```python
from build123d import *

# Parameters (mm, degrees)
SKETCH_1_W                    = 38
SKETCH_1_H                    = 78
EXTRUDE_1_DEPTH               = 7.8
SKETCH_3_W                    = 38
SKETCH_3_H                    = 7.8
EXTRUDE_2_DEPTH               = 78
EXTRUDE_3_DEPTH               = 3.8
SKETCH_5_R                    = 4.25
CUT_EXTRUDE_1_DEPTH           = 102.079572615
SKETCH_6_W                    = 8.8
SKETCH_6_H                    = 70
CUT_EXTRUDE_2_DEPTH           = 4
CUT_EXTRUDE_2_DRAFT           = -2
CUT_EXTRUDE_2_PROFILE_2_DEPTH = 4
CUT_EXTRUDE_2_PROFILE_2_DRAFT = -2
CUT_EXTRUDE_2_PROFILE_3_DEPTH = 4
CUT_EXTRUDE_2_PROFILE_3_DRAFT = -2
SKETCH_7_W                    = 8.8
SKETCH_7_H                    = 70
CUT_EXTRUDE_3_DEPTH           = 4
CUT_EXTRUDE_3_DRAFT           = -2
CUT_EXTRUDE_3_PROFILE_2_DEPTH = 4
CUT_EXTRUDE_3_PROFILE_2_DRAFT = -2
CUT_EXTRUDE_3_PROFILE_3_DEPTH = 4
CUT_EXTRUDE_3_PROFILE_3_DRAFT = -2


with BuildPart() as part:
    # 草图1 → 凸台-拉伸1 (new body)
    with BuildSketch(Plane.XY):
        Rectangle(SKETCH_1_W, SKETCH_1_H)
    extrude(amount=EXTRUDE_1_DEPTH)

    # 草图3 → 凸台-拉伸2 (add)
    with BuildSketch(Plane.XY.offset(7.8)):
        with Locations((0, -35.1)):
            Rectangle(SKETCH_3_W, SKETCH_3_H)
    extrude(amount=-EXTRUDE_2_DEPTH)

    # 草图4 → 凸台-拉伸3 (add)
    with BuildSketch(Plane.ZY.offset(19)):
        Polygon((0, 39), (-7.8, 39), (-7.8, 34), (-65.2, -23.4), (-70.2, -23.4), (-70.2, -31.2), (0, -31.2), align=None)
    extrude(amount=-EXTRUDE_3_DEPTH)

    # 草图5 → 切除-拉伸1 (cut, through all)
    with BuildSketch(Plane(origin=(0, -31.2, 0), x_dir=(1, 0, 0), z_dir=(0, 1, 0))):
        with Locations(Location((0, 54.416495981, 0), (0, 0, 270))):
            Circle(SKETCH_5_R)
        with BuildLine():
            Line((-4.1430597, 19.083232121), (-4.1430597, 36.583232121))
            ThreePointArc((-4.1430597, 36.583232121), (0, 40.726291822), (4.1430597, 36.583232121))
            Line((4.1430597, 36.583232121), (4.1430597, 19.083232121))
            ThreePointArc((4.1430597, 19.083232121), (0, 14.940172421), (-4.1430597, 19.083232121))
        make_face()
    cut_extrude_1 = extrude(amount=-CUT_EXTRUDE_1_DEPTH, mode=Mode.SUBTRACT)

    # 镜向1: 切除-拉伸1 across plane
    add(cut_extrude_1.mirror(Plane(origin=(0, -15.6, -15.6), x_dir=(0, -0.7071067811865478, 0.7071067811865474), z_dir=(0, 0.7071067811865472, 0.7071067811865478))), mode=Mode.SUBTRACT)


with BuildPart() as cut_extrude_2_tool:
    # 草图6 → 切除-拉伸2 (with draft: the straight prism first)
    with BuildSketch(Plane.XZ.offset(39)):
        with Locations((-11.8, -31.2)):
            Rectangle(SKETCH_6_W, SKETCH_6_H)
    extrude(amount=-CUT_EXTRUDE_2_DEPTH)
    # 切除-拉伸2: the draft: its side faces are tilted about the plane it starts from
    cut_extrude_2_sides = [cut_extrude_2_tool.faces().sort_by_distance(p)[0] for p in [
        (-16.2, -37, -31.2),
        (-11.8, -37, -66.2),
        (-7.4, -37, -31.2),
        (-11.8, -37, 3.8),
    ]]
    draft(cut_extrude_2_sides, Plane.XZ.offset(39), CUT_EXTRUDE_2_DRAFT)


with BuildPart() as part_1:
    add(part.part)

    # 切除-拉伸2: cut by cut_extrude_2_tool
    add(cut_extrude_2_tool.part, mode=Mode.SUBTRACT)


with BuildPart() as cut_extrude_2_profile_2_tool:
    # 草图6 → 切除-拉伸2 profile 2 (with draft: the straight prism first)
    with BuildSketch(Plane.XZ.offset(39)):
        with Locations((0, -31.2)):
            Rectangle(SKETCH_6_W, SKETCH_6_H)
    extrude(amount=-CUT_EXTRUDE_2_PROFILE_2_DEPTH)
    # 切除-拉伸2 profile 2: the draft: its side faces are tilted about the plane it starts from
    cut_extrude_2_profile_2_sides = [cut_extrude_2_profile_2_tool.faces().sort_by_distance(p)[0] for p in [
        (-4.4, -37, -31.2),
        (0, -37, -66.2),
        (4.4, -37, -31.2),
        (0, -37, 3.8),
    ]]
    draft(cut_extrude_2_profile_2_sides, Plane.XZ.offset(39), CUT_EXTRUDE_2_PROFILE_2_DRAFT)


with BuildPart() as part_2:
    add(part_1.part)

    # 切除-拉伸2 profile 2: cut by cut_extrude_2_profile_2_tool
    add(cut_extrude_2_profile_2_tool.part, mode=Mode.SUBTRACT)


with BuildPart() as cut_extrude_2_profile_3_tool:
    # 草图6 → 切除-拉伸2 profile 3 (with draft: the straight prism first)
    with BuildSketch(Plane.XZ.offset(39)):
        with Locations((11.8, -31.2)):
            Rectangle(SKETCH_6_W, SKETCH_6_H)
    extrude(amount=-CUT_EXTRUDE_2_PROFILE_3_DEPTH)
    # 切除-拉伸2 profile 3: the draft: its side faces are tilted about the plane it starts from
    cut_extrude_2_profile_3_sides = [cut_extrude_2_profile_3_tool.faces().sort_by_distance(p)[0] for p in [
        (7.4, -37, -31.2),
        (11.8, -37, -66.2),
        (16.2, -37, -31.2),
        (11.8, -37, 3.8),
    ]]
    draft(cut_extrude_2_profile_3_sides, Plane.XZ.offset(39), CUT_EXTRUDE_2_PROFILE_3_DRAFT)


with BuildPart() as part_3:
    add(part_2.part)

    # 切除-拉伸2 profile 3: cut by cut_extrude_2_profile_3_tool
    add(cut_extrude_2_profile_3_tool.part, mode=Mode.SUBTRACT)


with BuildPart() as cut_extrude_3_tool:
    # 草图7 → 切除-拉伸3 (with draft: the straight prism first)
    with BuildSketch(Plane.XY.offset(7.8)):
        Rectangle(SKETCH_7_W, SKETCH_7_H)
    extrude(amount=-CUT_EXTRUDE_3_DEPTH)
    # 切除-拉伸3: the draft: its side faces are tilted about the plane it starts from
    cut_extrude_3_sides = [cut_extrude_3_tool.faces().sort_by_distance(p)[0] for p in [
        (-4.4, 0, 5.8),
        (0, -35, 5.8),
        (4.4, 0, 5.8),
        (0, 35, 5.8),
    ]]
    draft(cut_extrude_3_sides, Plane.XY.offset(7.8), CUT_EXTRUDE_3_DRAFT)


with BuildPart() as part_4:
    add(part_3.part)

    # 切除-拉伸3: cut by cut_extrude_3_tool
    add(cut_extrude_3_tool.part, mode=Mode.SUBTRACT)


with BuildPart() as cut_extrude_3_profile_2_tool:
    # 草图7 → 切除-拉伸3 profile 2 (with draft: the straight prism first)
    with BuildSketch(Plane.XY.offset(7.8)):
        with Locations((-11.8, 0)):
            Rectangle(SKETCH_7_W, SKETCH_7_H)
    extrude(amount=-CUT_EXTRUDE_3_PROFILE_2_DEPTH)
    # 切除-拉伸3 profile 2: the draft: its side faces are tilted about the plane it starts from
    cut_extrude_3_profile_2_sides = [cut_extrude_3_profile_2_tool.faces().sort_by_distance(p)[0] for p in [
        (-16.2, 0, 5.8),
        (-11.8, -35, 5.8),
        (-7.4, 0, 5.8),
        (-11.8, 35, 5.8),
    ]]
    draft(cut_extrude_3_profile_2_sides, Plane.XY.offset(7.8), CUT_EXTRUDE_3_PROFILE_2_DRAFT)


with BuildPart() as part_5:
    add(part_4.part)

    # 切除-拉伸3 profile 2: cut by cut_extrude_3_profile_2_tool
    add(cut_extrude_3_profile_2_tool.part, mode=Mode.SUBTRACT)


with BuildPart() as cut_extrude_3_profile_3_tool:
    # 草图7 → 切除-拉伸3 profile 3 (with draft: the straight prism first)
    with BuildSketch(Plane.XY.offset(7.8)):
        with Locations((11.8, 0)):
            Rectangle(SKETCH_7_W, SKETCH_7_H)
    extrude(amount=-CUT_EXTRUDE_3_PROFILE_3_DEPTH)
    # 切除-拉伸3 profile 3: the draft: its side faces are tilted about the plane it starts from
    cut_extrude_3_profile_3_sides = [cut_extrude_3_profile_3_tool.faces().sort_by_distance(p)[0] for p in [
        (7.4, 0, 5.8),
        (11.8, -35, 5.8),
        (16.2, 0, 5.8),
        (11.8, 35, 5.8),
    ]]
    draft(cut_extrude_3_profile_3_sides, Plane.XY.offset(7.8), CUT_EXTRUDE_3_PROFILE_3_DRAFT)


with BuildPart() as part_6:
    add(part_5.part)

    # 切除-拉伸3 profile 3: cut by cut_extrude_3_profile_3_tool
    add(cut_extrude_3_profile_3_tool.part, mode=Mode.SUBTRACT)


solid = part_6.part
```
Part model, mm, in its own coordinate system. A direction names the side the tool comes from. Coordinates: 2 decimals unless noted, no trailing zeros. Write each loop counter-clockwise with the first axis right and the second up, starting at its lowest first coordinate (ties: lowest second). Pieces come first, ordered by that corner, then holes.
Item 1: Slice it at A-A (x = 0). Count the separate pieces of the cut face and the enclosed holes in it, and give its area (3 significant figures).
Item 2: Which spindle directions (+Z, -Z, +X, -X, +Y, -Y) get a long thin tool onto all of the face, cutting with end or side? Do faces 1 (the face through (4.143, -33, -28)), 2 (the face through (19, -32, -14)). Say none if no direction does.
Item 3: Slice it at C-C (z = -25). Write the cut outline in (x, y).
Item 4: Slice it at D-D (z = -2). Write the cut outline in (x, y), and give its area (3 significant figures).
Item 5: Pin check, flat tips, straight feed: pin 1 (9.5 mm diameter, centred on x = -10.5, y = -6.5, fed in from +Z); pin 2 (8 mm diameter, centred on x = -8.5, z = -15.5, fed in from +Y); pin 3 (2 mm diameter, centred on x = 3.5, y = 6, fed in from -Z); pin 4 (7.5 mm diameter, centred on x = 0, y = 23.22, fed in from -Z). Stop position of each tip, or through.
Item 6: Slice it at B-B (y = 2). Write the cut outline in (x, z), and give its area (3 significant figures).
Item 7: Probe line 1 (Y direction, x = 0, z = 1.3); line 2 (Y direction, x = 9, z = -9); line 3 (Z direction, x = 15, y = 3). List the from-to ranges inside material, lowest first.
Item 8: Mould opens along X. For faces 3 (the face through (-19, -8, -23)), 4 (the face through (4.143, -3, 2)), 5 (the face through (5, 4, 0)), 6 (the face through (-4.143, -33, -28)) say: released by +X, released by -X, zero draft, split by the parting line, or undercut.
Results found:
1. separate pieces: 5
1. enclosed holes: 0
1. area: 337 mm2
2. face 1: +Y, -Y
2. face 2: +Z, -Z, +X, +Y, -Y
3. outline: (-19, -39) - (-16.2, -39) - (-16.06, -35) - (-7.54, -35) - (-7.4, -39) - (-4.4, -39) - (-4.26, -35) - (-4.14, -35) - (-4.14, -31.2) - (-15.2, -31.2) - (-15.2, 16.8) - (-19, 16.8) - close; (4.14, -35) - (4.26, -35) - (4.4, -39) - (7.4, -39) - (7.54, -35) - (16.06, -35) - (16.2, -39) - (19, -39) - (19, -31.2) - (4.14, -31.2) - close
4. outline: (-19, -39) - (-16.2, -39) - (-16.06, -35) - (-7.54, -35) - (-7.4, -39) - (-4.4, -39) - (-4.26, -35) - (4.26, -35) - (4.4, -39) - (7.4, -39) - (7.54, -35) - (16.06, -35) - (16.2, -39) - (19, -39) - (19, -31.2) - (-15.2, -31.2) - (-15.2, 39) - (-19, 39) - close
4. area: 459 mm2
5. pin 1: stops at z = 7.8
5. pin 2: stops at y = -31.2
5. pin 3: stops at z = 0
5. pin 4: passes through
6. outline: (-19, -39.8) - (-15.2, -39.8) - (-15.2, 0) - (-4.14, 0) - (-4.14, 3.8) - (-4.26, 3.8) - (-4.4, 7.8) - (-7.4, 7.8) - (-7.54, 3.8) - (-16.06, 3.8) - (-16.2, 7.8) - (-19, 7.8) - close; (4.14, 0) - (19, 0) - (19, 7.8) - (16.2, 7.8) - (16.06, 3.8) - (7.54, 3.8) - (7.4, 7.8) - (4.4, 7.8) - (4.26, 3.8) - (4.14, 3.8) - close
6. area: 312 mm2
7. line 1: y = -35 to -16.26, 9.53 to 18.97, 27.47 to 39
7. line 2: y = -35 to -31.2
7. line 3: z = 0 to 3.8
8. face 3: released by -X
8. face 4: undercut
8. face 5: zero draft
8. face 6: undercut
